Work out the finished part from the listing and answer in its coordinate system (mm). Round coordinates to 2 decimals unless told otherwise and drop trailing zeros. Loops run counter-clockwise (first coordinate to the right, second up) from the corner with the lowest first, then second, coordinate; pieces in that order, holes last. Notation, with made-up numbers: (69, 72) -> (77, 72) arc R14 cw to (77, 97) -> close; hole circle Ø4 at (-7, 46). An arc over 180 degrees is marked (long way). Use CSV: the item, a comma, the result in double quotes. Start each with the question number.
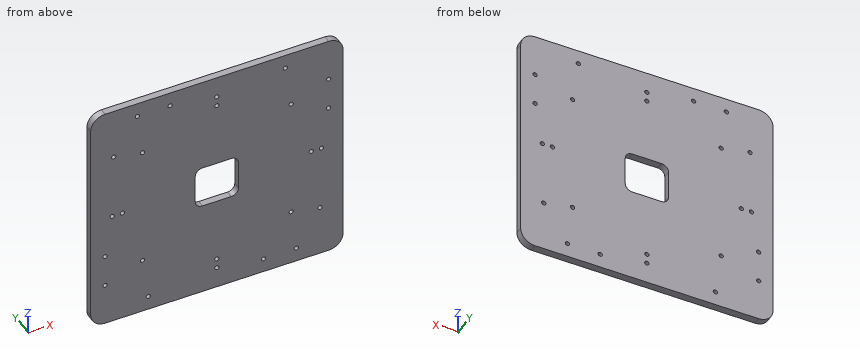
from build123d import *

# Parameters (mm, degrees)
RESSALTO_EXTRUS_O1_DEPTH = 5
ESBO_O2_R                = 1.5
CORTE_EXTRUS_O1_DEPTH    = 10
ESBO_O3_R                = 1.5
CORTE_EXTRUS_O2_DEPTH    = 15
ESBO_O4_R                = 1.5
CORTE_EXTRUS_O3_DEPTH    = 10
CORTE_EXTRUS_O4_DEPTH    = 10
ESBO_O6_R                = 1.5
CORTE_EXTRUS_O5_DEPTH    = 10


with BuildPart() as part:
    # Esboço1 → Ressalto-extrusão1 (new body)
    with BuildSketch(Plane(origin=(0, 0, 0), x_dir=(1, 0, 0), z_dir=(0, 1, 0))):
        with BuildLine():
            Line((-25.612995536, 137.664689841), (129.387004464, 137.664689841))
            ThreePointArc((129.387004464, 137.664689841), (136.458072276, 134.735757653), (139.387004464, 127.664689841))
            Line((139.387004464, 127.664689841), (139.387004464, -17.335310159))
            ThreePointArc((139.387004464, -17.335310159), (136.458072276, -24.406377971), (129.387004464, -27.335310159))
            Line((129.387004464, -27.335310159), (-25.612995536, -27.335310159))
            ThreePointArc((-25.612995536, -27.335310159), (-32.684063348, -24.406377971), (-35.612995536, -17.335310159))
            Line((-35.612995536, -17.335310159), (-35.612995536, 127.664689841))
            ThreePointArc((-35.612995536, 127.664689841), (-32.684063348, 134.735757653), (-25.612995536, 137.664689841))
        make_face()
    extrude(amount=RESSALTO_EXTRUS_O1_DEPTH)

    # Esboço2 → Corte-extrusão1 (cut)
    with BuildSketch(Plane(origin=(0, 5, 0), x_dir=(1, 0, 0), z_dir=(0, 1, 0))):
        with Locations(Location((0.387004464, 97.664689841, 0), (0, 0, 270))):
            Circle(ESBO_O2_R)
        with Locations(Location((103.387004464, 97.664689841, 0), (0, 0, 270))):
            Circle(ESBO_O2_R)
        with Locations(Location((0.387004464, 12.664689841, 0), (0, 0, 270))):
            Circle(ESBO_O2_R)
        with Locations(Location((103.387004464, 12.664689841, 0), (0, 0, 270))):
            Circle(ESBO_O2_R)
    extrude(amount=-CORTE_EXTRUS_O1_DEPTH, mode=Mode.SUBTRACT)

    # Esboço3 → Corte-extrusão2 (cut)
    with BuildSketch(Plane(origin=(0, 5, 0), x_dir=(1, 0, 0), z_dir=(0, 1, 0))):
        with Locations(Location((51.887004464, -5.335310159, 0), (0, 0, 270))):
            Circle(ESBO_O3_R)
        with Locations(Location((51.887004464, -12.335310159, 0), (0, 0, 270))):
            Circle(ESBO_O3_R)
        with Locations(Location((-20.612995536, 55.164689841, 0), (0, 0, 270))):
            Circle(ESBO_O3_R)
        with Locations(Location((-13.612995536, 55.164689841, 0), (0, 0, 270))):
            Circle(ESBO_O3_R)
        with Locations(Location((51.887004464, 122.664689841, 0), (0, 0, 90))):
            Circle(ESBO_O3_R)
        with Locations(Location((51.887004464, 115.664689841, 0), (0, 0, 90))):
            Circle(ESBO_O3_R)
        with Locations(Location((124.387004464, 55.164689841, 0), (0, 0, 90))):
            Circle(ESBO_O3_R)
        with Locations(Location((117.387004464, 55.164689841, 0), (0, 0, 90))):
            Circle(ESBO_O3_R)
    extrude(amount=-CORTE_EXTRUS_O2_DEPTH, mode=Mode.SUBTRACT)

    # Esboço4 → Corte-extrusão3 (cut)
    with BuildSketch(Plane(origin=(0, 5, 0), x_dir=(1, 0, 0), z_dir=(0, 1, 0))):
        with Locations(Location((-3.212995536, -17.335310159, 0), (0, 0, 270))):
            Circle(ESBO_O4_R)
        with Locations(Location((19.487004464, -17.335310159, 0), (0, 0, 270))):
            Circle(ESBO_O4_R)
        with Locations(Location((-25.612995536, 107.764689841, 0), (0, 0, 270))):
            Circle(ESBO_O4_R)
        with Locations(Location((-25.612995536, 85.064689841, 0), (0, 0, 270))):
            Circle(ESBO_O4_R)
        with Locations(Location((106.987004464, 127.664689841, 0), (0, 0, 270))):
            Circle(ESBO_O4_R)
        with Locations(Location((84.287004464, 127.664689841, 0), (0, 0, 270))):
            Circle(ESBO_O4_R)
        with Locations(Location((129.387004464, 2.564689841, 0), (0, 0, 270))):
            Circle(ESBO_O4_R)
        with Locations(Location((129.387004464, 25.264689841, 0), (0, 0, 270))):
            Circle(ESBO_O4_R)
    extrude(amount=-CORTE_EXTRUS_O3_DEPTH, mode=Mode.SUBTRACT)

    # Esboço5 → Corte-extrusão4 (cut)
    with BuildSketch(Plane(origin=(0, 5, 0), x_dir=(1, 0, 0), z_dir=(0, 1, 0))):
        with BuildLine():
            Line((41.887004464, 40.164689841), (61.887004464, 40.164689841))
            ThreePointArc((61.887004464, 40.164689841), (65.42253837, 41.629155935), (66.887004464, 45.164689841))
            Line((66.887004464, 45.164689841), (66.887004464, 65.164689841))
            ThreePointArc((66.887004464, 65.164689841), (65.42253837, 68.700223747), (61.887004464, 70.164689841))
            Line((61.887004464, 70.164689841), (41.887004464, 70.164689841))
            ThreePointArc((41.887004464, 70.164689841), (38.351470558, 68.700223747), (36.887004464, 65.164689841))
            Line((36.887004464, 65.164689841), (36.887004464, 45.164689841))
            ThreePointArc((36.887004464, 45.164689841), (38.351470558, 41.629155935), (41.887004464, 40.164689841))
        make_face()
    extrude(amount=-CORTE_EXTRUS_O4_DEPTH, mode=Mode.SUBTRACT)

    # Esboço6 → Corte-extrusão5 (cut)
    with BuildSketch(Plane(origin=(0, 5, 0), x_dir=(1, 0, 0), z_dir=(0, 1, 0))):
        with Locations(Location((-19.612995536, 8.664689841, 0), (0, 0, 270))):
            Circle(ESBO_O6_R)
        with Locations(Location((123.387004464, 101.664689841, 0), (0, 0, 270))):
            Circle(ESBO_O6_R)
        with Locations(Location((4.387004464, 127.664689841, 0), (0, 0, 270))):
            Circle(ESBO_O6_R)
        with Locations(Location((99.387004464, -17.335310159, 0), (0, 0, 270))):
            Circle(ESBO_O6_R)
    extrude(amount=-CORTE_EXTRUS_O5_DEPTH, mode=Mode.SUBTRACT)


solid = part.part
Q1. Each of these flat-tipped pins is pushed along its axis until it touches: pin 1 (1.8 mm diameter, centred on x = 103.39, z = -97.66, fed in from -Y); pin 2 (5 mm diameter, centred on x = 103.39, z = -12.66, fed in from -Y). Where does it stop, or does it pass through?
Q2. Section B-B, the plane y = 2.6 is taken. Give the number of separate pieces and of enclosed holes in the cut face, and give its area (3 significant figures).
Q3. Straight lines are drawn through the part: line 1 (Z direction, x = 129.5, y = 3.15); line 2 (Z direction, x = 123.5, y = 0.2); line 3 (X direction, y = 1.35, z = -51). For each, find the intervals that lie inside material, in ascending order. Write a range as from..to.
Q4. Section A-A, the plane x = 44 is taken. Write down the section's boundary in (y, z).
Report:
1,pin 1,"passes through"
1,pin 2,"stops at y = 0"
2,separate pieces,"1"
2,enclosed holes,"25"
2,area,"27,700 mm²"
3,line 1,"z = -137.66..-26.76, -23.77..-4.06, -1.07..27.33"
3,line 2,"z = -137.66..-103.16, -100.17..-56.37, -53.96..27.34"
3,line 3,"x = -35.61..36.89, 66.89..139.39"
4,outline,"(0, -137.66) -> (5, -137.66) -> (5, -70.16) -> (0, -70.16) -> close; (0, -40.16) -> (5, -40.16) -> (5, 27.34) -> (0, 27.34) -> close"
